Part model, mm, in its own coordinate system. Coordinates: 2 decimals unless noted, no trailing zeros. Order: outer loops, then holes, each group sorted by start corner. A loop starts at its lowest first (then second) coordinate and runs counter-clockwise, first axis right, second up.
from build123d import *

# Parameters (mm, degrees)
SKETCH_1_W      = 130
SKETCH_1_H      = 200
SKETCH_1_R      = 1.75
SKETCH_1_R_2    = 2.25
SKETCH_1_R_3    = 2
EXTRUDE_2_DEPTH = 3
FILLET_1_R      = 20
FILLET_2_R      = 20
FILLET_3_R      = 20
FILLET_4_R      = 20


with BuildPart() as part:
    # 草图1 → 凸台-拉伸2 (new body)
    with BuildSketch(Plane(origin=(0, 0, 0), x_dir=(1, 0, 0), z_dir=(0, 1, 0))):
        Rectangle(SKETCH_1_W, SKETCH_1_H)
        with Locations((52, -70)):
            Circle(SKETCH_1_R, mode=Mode.SUBTRACT)
        with Locations((52, -40)):
            Circle(SKETCH_1_R, mode=Mode.SUBTRACT)
        with Locations((28, -40)):
            Circle(SKETCH_1_R, mode=Mode.SUBTRACT)
        with Locations((28, -70)):
            Circle(SKETCH_1_R, mode=Mode.SUBTRACT)
        with Locations((52, 40)):
            Circle(SKETCH_1_R, mode=Mode.SUBTRACT)
        with Locations((52, 70)):
            Circle(SKETCH_1_R, mode=Mode.SUBTRACT)
        with Locations((28, 70)):
            Circle(SKETCH_1_R, mode=Mode.SUBTRACT)
        with Locations((28, 40)):
            Circle(SKETCH_1_R, mode=Mode.SUBTRACT)
        with Locations((-28, 40)):
            Circle(SKETCH_1_R, mode=Mode.SUBTRACT)
        with Locations((-28, 70)):
            Circle(SKETCH_1_R, mode=Mode.SUBTRACT)
        with Locations((-52, 70)):
            Circle(SKETCH_1_R, mode=Mode.SUBTRACT)
        with Locations((-52, 40)):
            Circle(SKETCH_1_R, mode=Mode.SUBTRACT)
        with Locations((-28, -70)):
            Circle(SKETCH_1_R, mode=Mode.SUBTRACT)
        with Locations((-28, -40)):
            Circle(SKETCH_1_R, mode=Mode.SUBTRACT)
        with Locations((-52, -40)):
            Circle(SKETCH_1_R, mode=Mode.SUBTRACT)
        with Locations((-52, -70)):
            Circle(SKETCH_1_R, mode=Mode.SUBTRACT)
        with Locations((35, -35)):
            Circle(SKETCH_1_R_2, mode=Mode.SUBTRACT)
        with Locations((-35, -35)):
            Circle(SKETCH_1_R_2, mode=Mode.SUBTRACT)
        with Locations((-35, 35)):
            Circle(SKETCH_1_R_2, mode=Mode.SUBTRACT)
        with Locations((35, 35)):
            Circle(SKETCH_1_R_2, mode=Mode.SUBTRACT)
        with Locations((16, 90)):
            Circle(SKETCH_1_R, mode=Mode.SUBTRACT)
        with Locations((-16, 90)):
            Circle(SKETCH_1_R, mode=Mode.SUBTRACT)
        with Locations((-34.5, 90)):
            Circle(SKETCH_1_R, mode=Mode.SUBTRACT)
        with Locations((34.5, 90)):
            Circle(SKETCH_1_R, mode=Mode.SUBTRACT)
        with Locations((-8, 73)):
            Circle(SKETCH_1_R, mode=Mode.SUBTRACT)
        with Locations((0, 65)):
            Circle(SKETCH_1_R, mode=Mode.SUBTRACT)
        with Locations((0, 81)):
            Circle(SKETCH_1_R, mode=Mode.SUBTRACT)
        with Locations((8, 73)):
            Circle(SKETCH_1_R, mode=Mode.SUBTRACT)
        with Locations((-8, -73)):
            Circle(SKETCH_1_R, mode=Mode.SUBTRACT)
        with Locations((0, -81)):
            Circle(SKETCH_1_R, mode=Mode.SUBTRACT)
        with Locations((0, -65)):
            Circle(SKETCH_1_R, mode=Mode.SUBTRACT)
        with Locations((8, -73)):
            Circle(SKETCH_1_R, mode=Mode.SUBTRACT)
        with Locations((15, 45)):
            Circle(SKETCH_1_R_3, mode=Mode.SUBTRACT)
        with Locations((-15, 45)):
            Circle(SKETCH_1_R_3, mode=Mode.SUBTRACT)
        with Locations((-15, 68)):
            Circle(SKETCH_1_R_3, mode=Mode.SUBTRACT)
        with Locations((15, 68)):
            Circle(SKETCH_1_R_3, mode=Mode.SUBTRACT)
        with Locations((15, -68)):
            Circle(SKETCH_1_R_3, mode=Mode.SUBTRACT)
        with Locations((-15, -68)):
            Circle(SKETCH_1_R_3, mode=Mode.SUBTRACT)
        with Locations((-15, -45)):
            Circle(SKETCH_1_R_3, mode=Mode.SUBTRACT)
        with Locations((15, -45)):
            Circle(SKETCH_1_R_3, mode=Mode.SUBTRACT)
        with Locations((35, 85)):
            Circle(SKETCH_1_R_3, mode=Mode.SUBTRACT)
        with Locations((-35, 85)):
            Circle(SKETCH_1_R_3, mode=Mode.SUBTRACT)
        with Locations((35, -85)):
            Circle(SKETCH_1_R_3, mode=Mode.SUBTRACT)
        with Locations((-35, -85)):
            Circle(SKETCH_1_R_3, mode=Mode.SUBTRACT)
        with Locations((8, -58)):
            Circle(SKETCH_1_R_3, mode=Mode.SUBTRACT)
        with Locations((8, -95)):
            Circle(SKETCH_1_R_3, mode=Mode.SUBTRACT)
        with Locations((45, -95)):
            Circle(SKETCH_1_R_3, mode=Mode.SUBTRACT)
        with Locations((-45, -95)):
            Circle(SKETCH_1_R_3, mode=Mode.SUBTRACT)
        with Locations((-8, -95)):
            Circle(SKETCH_1_R_3, mode=Mode.SUBTRACT)
        with Locations((-8, -58)):
            Circle(SKETCH_1_R_3, mode=Mode.SUBTRACT)
        with Locations((45, 95)):
            Circle(SKETCH_1_R_3, mode=Mode.SUBTRACT)
        with Locations((8, 95)):
            Circle(SKETCH_1_R_3, mode=Mode.SUBTRACT)
        with Locations((-8, 95)):
            Circle(SKETCH_1_R_3, mode=Mode.SUBTRACT)
        with Locations((-45, 95)):
            Circle(SKETCH_1_R_3, mode=Mode.SUBTRACT)
        with Locations((8, 58)):
            Circle(SKETCH_1_R_3, mode=Mode.SUBTRACT)
        with Locations((-8, 58)):
            Circle(SKETCH_1_R_3, mode=Mode.SUBTRACT)
        with Locations((19.5, -56.5)):
            Circle(SKETCH_1_R_3, mode=Mode.SUBTRACT)
        with Locations((-19.5, -56.5)):
            Circle(SKETCH_1_R_3, mode=Mode.SUBTRACT)
        with Locations((-19.5, 56.5)):
            Circle(SKETCH_1_R_3, mode=Mode.SUBTRACT)
        with Locations((19.5, 56.5)):
            Circle(SKETCH_1_R_3, mode=Mode.SUBTRACT)
        with BuildLine():
            Line((-40, -88.25), (40, -88.25))
            ThreePointArc((40, -88.25), (41.75, -90), (40, -91.75))
            Line((40, -91.75), (-40, -91.75))
            ThreePointArc((-40, -91.75), (-41.75, -90), (-40, -88.25))
        make_face(mode=Mode.SUBTRACT)
        with BuildLine():
            Line((42.5, -20), (42.5, 20))
            ThreePointArc((42.5, 20), (50, 27.5), (57.5, 20))
            Line((57.5, 20), (57.5, -20))
            ThreePointArc((57.5, -20), (50, -27.5), (42.5, -20))
        make_face(mode=Mode.SUBTRACT)
        with BuildLine():
            Line((-57.5, -20), (-57.5, 20))
            ThreePointArc((-57.5, 20), (-50, 27.5), (-42.5, 20))
            Line((-42.5, 20), (-42.5, -20))
            ThreePointArc((-42.5, -20), (-50, -27.5), (-57.5, -20))
        make_face(mode=Mode.SUBTRACT)
    extrude(amount=EXTRUDE_2_DEPTH)

    # 圆角1
    fillet_1_edges = [part.edges().sort_by_distance(p)[0] for p in [
        (65, 1.5, 100),
    ]]
    fillet(fillet_1_edges, radius=FILLET_1_R)

    # 圆角2
    fillet_2_edges = [part.edges().sort_by_distance(p)[0] for p in [
        (-65, 1.5, 100),
    ]]
    fillet(fillet_2_edges, radius=FILLET_2_R)

    # 圆角3
    fillet_3_edges = [part.edges().sort_by_distance(p)[0] for p in [
        (-65, 1.5, -100),
    ]]
    fillet(fillet_3_edges, radius=FILLET_3_R)

    # 圆角4
    fillet_4_edges = [part.edges().sort_by_distance(p)[0] for p in [
        (65, 1.5, -100),
    ]]
    fillet(fillet_4_edges, radius=FILLET_4_R)


solid = part.part
Q1. Cut at B-B on y = 2.2. Count the separate pieces of the cut face and the enclosed holes in it, and give its area (3 significant figures).
Results list:
separate pieces: 1
enclosed holes: 63
area: 23,100 mm2
Q2. Mould opens along X. For faces 1 (the face through (58.986, 1.521, -94.297)), 2 (the face through (36.21, 1.479, -36.897)) say: pulls with the +X half, pulls with the -X half, needs draft (parallel to the pull), parting line crosses it, or undercut.
Results list:
face 1: pulls with the +X half
face 2: undercut
Q3. Cut at A-A on z = 5. Write the cut outline in (x, y).
Results list:
outline: (-65, 0) - (-57.5, 0) - (-57.5, 3) - (-65, 3) - close; (-42.5, 0) - (42.5, 0) - (42.5, 3) - (-42.5, 3) - close; (57.5, 0) - (65, 0) - (65, 3) - (57.5, 3) - close
Q4. Wall check: line 1 along Z through (x, y) = (0, 1.5); line 2 along X through (y, z) = (0.75, -17); line 3 along X through (y, z) = (1.15, -40). Give the ranges that are in metal, low to high.
Results list:
line 1: z = -100 to -82.75, -79.25 to -66.75, -63.25 to 63.25, 66.75 to 79.25, 82.75 to 88.25, 91.75 to 100
line 2: x = -65 to -57.5, -42.5 to 42.5, 57.5 to 65
line 3: x = -65 to -53.75, -50.25 to -29.75, -26.25 to 26.25, 29.75 to 50.25, 53.75 to 65
